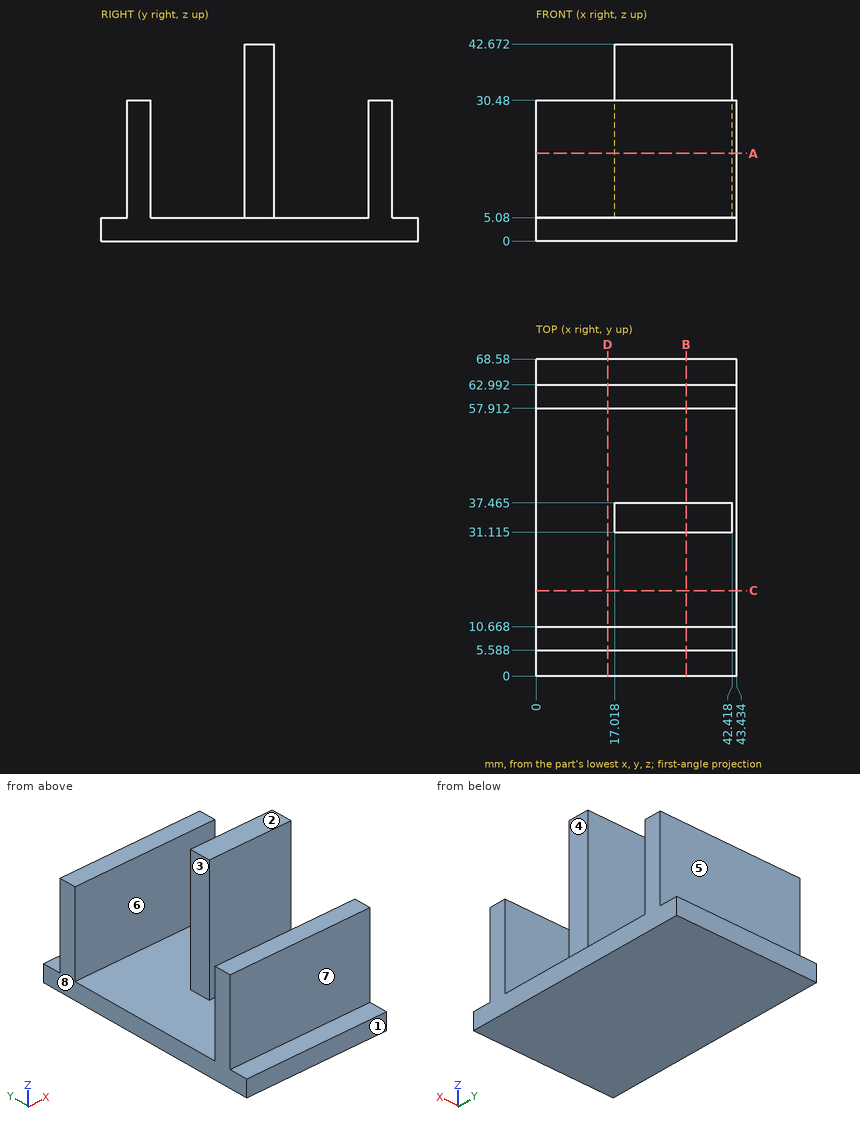
Can you work these out from the drawing? Everything is in mm from the part's minimum corner. A direction names the side the tool comes from. Give positions to 0.01 mm unless a question says otherwise; leave off trailing zeros. Write each loop counter-clockwise with the first axis right and the second up, starting at its lowest first coordinate (ties: lowest second). Pieces come first, ordered by that corner, then holes. Notation, with made-up numbers: M 67,29.25 L 107,29.25 A9 cw 107,38.25 Z; hole C 45.5,-9.75 d7. An arc over 180 degrees is marked long. Answer in a Markdown table with one row per item. Add a question column.
Item 1: Imagine slicing it at B-B, the plane x = 32.5. Write out the boundary of the cut face in (y, z) (3 decimals).
Item 2: On a 3-axis mill with a long thin cutter (end or side, diameter ignored), from which of +Z, -Z, +X, -X, +Y, -Y can I reach the whole of each face in a straight line? I mean the marked faces 4, 5, 6, 7 and 8. Say none if no direction works.
Item 3: We'd pull the mould along Y, two halves only. Please class the marked faces 1, 2 and 3: released by +Y, released by -Y, zero draft, split by the parting line, or undercut.
Item 4: Imagine slicing it at D-D, the plane x = 15.5. Write out the boundary of the cut face in (y, z).
Item 5: Please list where these lines run through material, in increasing order: L1, parallel to Y at x = 33.5, z = 16 (3 decimals); L2, parallel to Y at x = 9.5, z = 24.5; L3, parallel to Z at x = 11, y = 31.5.
Item 6: Imagine slicing it at C-C, the plane y = 18.5. Write out the boundary of the cut face in (x, z), plus the area to 3 significant figures.
Item 7: Imagine slicing it at A-A, the plane z = 19. Write out the boundary of the cut face in (x, y) (3 decimals).
Item 8: For pin 1 Ø5.5 at (x, y) = (23, 59.5) entering from +Z; pin 2 Ø7.5 at (x, z) = (29, 15) entering from -Y; pin 3 Ø10 at (x, z) = (21, 10.5) entering from +Y, each with a flat end and sliding along its axis, tell me the tip position at first contact or that it passes through.
Evaluation:
| question | item | result |
|---|---|---|
| 1 | outline | M 0,0 L 68.58,0 L 68.58,5.08 L 62.992,5.08 L 62.992,30.48 L 57.912,30.48 L 57.912,5.08 L 37.465,5.08 L 37.465,42.672 L 31.115,42.672 L 31.115,5.08 L 10.668,5.08 L 10.668,30.48 L 5.588,30.48 L 5.588,5.08 L 0,5.08 Z |
| 2 | face 4 | +Z, +X |
| 2 | face 5 | +Z, +X, -X, +Y |
| 2 | face 6 | +Z, +X, -X |
| 2 | face 7 | +Z, +X, -X, -Y |
| 2 | face 8 | +Z, -Z, -X, +Y, -Y |
| 3 | face 1 | released by -Y |
| 3 | face 2 | zero draft |
| 3 | face 3 | undercut |
| 4 | outline | M 0,0 L 68.58,0 L 68.58,5.08 L 62.99,5.08 L 62.99,30.48 L 57.91,30.48 L 57.91,5.08 L 10.67,5.08 L 10.67,30.48 L 5.59,30.48 L 5.59,5.08 L 0,5.08 Z |
| 5 | L1 | y = 5.588 to 10.668, 31.115 to 37.465, 57.912 to 62.992 |
| 5 | L2 | y = 5.59 to 10.67, 57.91 to 62.99 |
| 5 | L3 | z = 0 to 5.08 |
| 6 | outline | M 0,0 L 43.43,0 L 43.43,5.08 L 0,5.08 Z |
| 6 | area | 221 mm² |
| 7 | outline | M 0,5.588 L 43.434,5.588 L 43.434,10.668 L 0,10.668 Z; M 0,57.912 L 43.434,57.912 L 43.434,62.992 L 0,62.992 Z; M 17.018,31.115 L 42.418,31.115 L 42.418,37.465 L 17.018,37.465 Z |
| 8 | pin 1 | stops at z = 30.48 |
| 8 | pin 2 | stops at y = 5.59 |
| 8 | pin 3 | stops at y = 62.99 |
